Work out the finished part from the listing and answer in its coordinate system (mm). A direction names the side the tool comes from. Give positions to 0.01 mm unless a question says otherwise; leave off trailing zeros. Loops run counter-clockwise (first coordinate to the right, second up) from the corner with the lowest first, then second, coordinate; pieces in that order, holes last. Notation, with made-up numbers: M 51.25,13 L 65.25,13 A13 cw 65.25,36 Z; hole C 82.25,-33 d2. An arc over 180 degrees is marked long. Answer in a Markdown table with one row per item. Add a question column.
from build123d import *

# Parameters (mm, degrees)
SKETCH1_W                  = 40
SKETCH1_H                  = 25
BOSS_EXTRUDE1_DEPTH        = 2
SKETCH2_W                  = 5
SKETCH2_H                  = 20
BOSS_EXTRUDE2_DEPTH        = 10
SKETCH4_W                  = 19.965035534
SKETCH4_H                  = 6
BOSS_EXTRUDE3_DEPTH        = 5
SKETCH5_R                  = 1
CUT_EXTRUDE2_DEPTH         = 5
SKETCH6_W                  = 4
SKETCH6_H                  = 5
BOSS_EXTRUDE4_DEPTH        = 10
SKETCH8_W                  = 5
SKETCH8_H                  = 4
BOSS_EXTRUDE5_DEPTH        = 10
SKETCH9_W                  = 4
SKETCH9_H                  = 5
BOSS_EXTRUDE6_DEPTH        = 45
SKETCH12_W                 = 18
SKETCH12_H                 = 4
BOSS_EXTRUDE8_DEPTH        = 4
SKETCH13_W                 = 5
SKETCH13_H                 = 4
BOSS_EXTRUDE9_DEPTH        = 26
SKETCH14_W                 = 18
SKETCH14_H                 = 4
BOSS_EXTRUDE10_DEPTH       = 6
SKETCH16_W                 = 5.988277512
SKETCH16_H                 = 18
BOSS_EXTRUDE11_DEPTH       = 5
SKETCH15_R                 = 1
CUT_EXTRUDE3_DEPTH         = 6
SKETCH17_R                 = 3
CUT_EXTRUDE5_DEPTH         = 6
SKETCH24_W                 = 8
SKETCH24_H                 = 18.5
BOSS_EXTRUDE18_DEPTH       = 4
BOSS_EXTRUDE20_START       = -1
SKETCH20_R                 = 5
SKETCH20_R_2               = 3
BOSS_EXTRUDE20_DEPTH       = 1
BOSS_EXTRUDE21_OUTLINE_R   = 2.998308623
BOSS_EXTRUDE21_OUTLINE_R_2 = 1.5
BOSS_EXTRUDE21_DEPTH       = 1
SKETCH27_R                 = 5
SKETCH27_R_2               = 2.75
BOSS_EXTRUDE22_DEPTH       = 2
SKETCH28_R                 = 2.75
CUT_EXTRUDE10_DEPTH        = 10
SKETCH29_R                 = 5
BOSS_EXTRUDE23_DEPTH       = 5


# Read off the part's stored shape, not the designer's step: Boss-Extrude21
with BuildPart() as part:
    # Sketch1 → Boss-Extrude1 (new body)
    with BuildSketch(Plane(origin=(0, 0, 0), x_dir=(1, 0, 0), z_dir=(0, 1, 0))):
        Rectangle(SKETCH1_W, SKETCH1_H)
    extrude(amount=BOSS_EXTRUDE1_DEPTH)

    # Sketch2 → Boss-Extrude2 (add)
    with BuildSketch(Plane(origin=(0, 2, 0), x_dir=(1, 0, 0), z_dir=(0, 1, 0))):
        with Locations((4.5, 0)):
            Rectangle(SKETCH2_W, SKETCH2_H)
    extrude(amount=BOSS_EXTRUDE2_DEPTH)

    # Sketch4 → Boss-Extrude3 (add)
    with BuildSketch(Plane(origin=(7, 0, 0), x_dir=(0, 0, -1), z_dir=(1, 0, 0))):
        with Locations((-0.017482233, 9)):
            Rectangle(SKETCH4_W, SKETCH4_H)
    extrude(amount=-BOSS_EXTRUDE3_DEPTH)

    # Sketch5 → Cut-Extrude2 (cut)
    with BuildSketch(Plane(origin=(7, 0, 0), x_dir=(0, 0, -1), z_dir=(1, 0, 0))):
        with Locations((5, 7.5)):
            Circle(SKETCH5_R)
        with Locations((-5, 7.5)):
            Circle(SKETCH5_R)
    extrude(amount=-CUT_EXTRUDE2_DEPTH, mode=Mode.SUBTRACT)

    # Sketch6 → Boss-Extrude4 (add)
    with BuildSketch(Plane(origin=(0, 2, 0), x_dir=(1, 0, 0), z_dir=(0, 1, 0))):
        with Locations((-11.527661753, -6.5)):
            Rectangle(SKETCH6_W, SKETCH6_H)
        with Locations((-11.527661753, 6.5)):
            Rectangle(SKETCH6_W, SKETCH6_H)
    extrude(amount=BOSS_EXTRUDE4_DEPTH)

    # Sketch8 → Boss-Extrude5 (add)
    with BuildSketch(Plane.ZY.offset(13.527661753)):
        with Locations((-6.5, 10)):
            Rectangle(SKETCH8_W, SKETCH8_H)
    boss_extrude5 = extrude(amount=BOSS_EXTRUDE5_DEPTH)

    # Mirror1: Boss-Extrude5 across plane
    add(boss_extrude5.mirror(Plane(origin=(0, 0, 0), x_dir=(1, 0, 0), z_dir=(0, 0, -1))))

    # Sketch9 → Boss-Extrude6 (add)
    with BuildSketch(Plane(origin=(0, 12, 0), x_dir=(1, 0, 0), z_dir=(0, 1, 0))):
        with Locations((-21.527661753, 6.5)):
            Rectangle(SKETCH9_W, SKETCH9_H)
    boss_extrude6 = extrude(amount=BOSS_EXTRUDE6_DEPTH)

    # Mirror2: Boss-Extrude5 across plane
    add(boss_extrude5.mirror(Plane(origin=(0, 0, 0), x_dir=(1, 0, 0), z_dir=(0, 0, -1))))

    # Mirror3: Boss-Extrude6 across plane
    add(boss_extrude6.mirror(Plane(origin=(0, 0, 0), x_dir=(1, 0, 0), z_dir=(0, 0, -1))))

    # Sketch12 → Boss-Extrude8 (add)
    with BuildSketch(Plane.ZY.offset(23.527661753)):
        with Locations((0, 55)):
            Rectangle(SKETCH12_W, SKETCH12_H)
        with Locations((0, 10)):
            Rectangle(SKETCH12_W, SKETCH12_H)
        with Locations((0, 32.5)):
            Rectangle(SKETCH12_W, SKETCH12_H)
    extrude(amount=-BOSS_EXTRUDE8_DEPTH)

    # Sketch13 → Boss-Extrude9 (add)
    with BuildSketch(Plane(origin=(-19.527661753, 0, 0), x_dir=(0, 0, -1), z_dir=(1, 0, 0))):
        with Locations((-6.5, 55)):
            Rectangle(SKETCH13_W, SKETCH13_H)
        with Locations((6.5, 55)):
            Rectangle(SKETCH13_W, SKETCH13_H)
    extrude(amount=BOSS_EXTRUDE9_DEPTH)

    # Sketch14 → Boss-Extrude10 (add)
    with BuildSketch(Plane(origin=(6.472338247, 0, 0), x_dir=(0, 0, -1), z_dir=(1, 0, 0))):
        with Locations((0, 55)):
            Rectangle(SKETCH14_W, SKETCH14_H)
    extrude(amount=-BOSS_EXTRUDE10_DEPTH)

    # Sketch16 → Boss-Extrude11 (add)
    with BuildSketch(Plane(origin=(0, 57, 0), x_dir=(1, 0, 0), z_dir=(0, 1, 0))):
        with Locations((3.478199491, 0)):
            Rectangle(SKETCH16_W, SKETCH16_H)
    extrude(amount=BOSS_EXTRUDE11_DEPTH)

    # Sketch15 → Cut-Extrude3 (cut)
    with BuildSketch(Plane(origin=(6.472338247, 0, 0), x_dir=(0, 0, -1), z_dir=(1, 0, 0))):
        with Locations((-5, 57.5)):
            Circle(SKETCH15_R)
        with Locations((5, 57.5)):
            Circle(SKETCH15_R)
    extrude(amount=-CUT_EXTRUDE3_DEPTH, mode=Mode.SUBTRACT)

    # Sketch17 → Cut-Extrude5 (cut)
    with BuildSketch(Plane.XZ):
        with Locations(Location((0, 0, 0), (0, 0, 270))):
            Circle(SKETCH17_R)
    extrude(amount=-CUT_EXTRUDE5_DEPTH, mode=Mode.SUBTRACT)

    # Sketch24 → Boss-Extrude18 (add)
    with BuildSketch(Plane.ZY.offset(23.527661753)):
        with Locations((0, 43.75)):
            Rectangle(SKETCH24_W, SKETCH24_H)
    extrude(amount=-BOSS_EXTRUDE18_DEPTH)

    # Sketch20 → Boss-Extrude20 (add)
    with BuildSketch(Plane(origin=(0, 3, 0), x_dir=(1, 0, 0), z_dir=(0, 1, 0)).offset(BOSS_EXTRUDE20_START)):
        Circle(SKETCH20_R)
        with Locations(Location((0, 0, 0), (0, 0, 90))):
            Circle(SKETCH20_R_2, mode=Mode.SUBTRACT)
    extrude(amount=BOSS_EXTRUDE20_DEPTH)

    # Boss-Extrude21 outline → Boss-Extrude21 (add)
    # profile 1 of 2: a face of its own
    with BuildSketch(Plane(origin=(0, 3, 0), x_dir=(1, 0, 0), z_dir=(0, 1, 0))):
        with BuildLine():
            ThreePointArc((2, -2.236067977), (-3, 0), (2, 2.236067977))
            Line((2, 2.236067977), (2, 4.582575695))
            ThreePointArc((2, 4.582575695), (-5, 0), (2, -4.582575695))
            Line((2, -4.582575695), (2, -2.236067977))
        make_face()
    # profile 2 of 2: a face of its own
    with BuildSketch(Plane(origin=(0, 3, 0), x_dir=(1, 0, 0), z_dir=(0, 1, 0))):
        Circle(BOSS_EXTRUDE21_OUTLINE_R)
        Circle(BOSS_EXTRUDE21_OUTLINE_R_2, mode=Mode.SUBTRACT)
    extrude(amount=BOSS_EXTRUDE21_DEPTH)

    # Sketch27 → Boss-Extrude22 (add)
    with BuildSketch(Plane(origin=(0, 4, 0), x_dir=(1, 0, 0), z_dir=(0, 1, 0))):
        Circle(SKETCH27_R)
        with Locations(Location((0, 0, 0), (0, 0, 43.341758227))):
            Circle(SKETCH27_R_2, mode=Mode.SUBTRACT)
    extrude(amount=BOSS_EXTRUDE22_DEPTH)

    # Sketch28 → Cut-Extrude10 (cut)
    with BuildSketch(Plane(origin=(0, 6, 0), x_dir=(1, 0, 0), z_dir=(0, 1, 0))):
        with Locations(Location((0, 0, 0), (0, 0, 43.341758227))):
            Circle(SKETCH28_R)
    extrude(amount=CUT_EXTRUDE10_DEPTH, mode=Mode.SUBTRACT)

    # Sketch29 → Boss-Extrude23 (add)
    with BuildSketch(Plane.ZY.offset(23.527661753)):
        with Locations((-0.05, 43.4)):
            Circle(SKETCH29_R)
    extrude(amount=BOSS_EXTRUDE23_DEPTH)


solid = part.part
(1) Each of these flat-tipped pins is pushed along its axis until it touches: P1, Ø2.5, axis at y = 4, z = 6.5, coming from the -X side; P2, Ø1, axis at y = 36.5, z = 2.5, coming from the +X side; P3, Ø1.6, axis at y = 57.5, z = -5, coming from the +X side. Where does it stop, or does it pass through?
(2) Section B-B, the plane z = 7 is taken. Determine the outline of the cut face in (x, y).
(3) The mould has two halves that part along Y. Classify faces 1 (the face through (1.3, 3, 1.3)), 2 (the face through (-13, 8, 4)), 3 (the face through (-25.99, 38.52, -1.13)), 4 (the face through (4.54, 8.49, -4.87)): pulls with the +Y half, pulls with the -Y half, needs draft (parallel to the pull), parting line crosses it, or undercut.
(4) Section D-D, the plane y = 37.5 is taken. Determine the outline of the cut face in (x, z), and give its area (3 significant figures).
(5) Section A-A, the plane y = 10.5 is taken. Determine the outline of the cut face in (x, z).
(6) Section C-C, the plane x = -24.5 is taken. Determine the outline of the cut face in (y, z).
(7) Which of the six approach directions +Z, -Z, +X, -X, +Y, -Y give full straight-line access (tool end or side, diameter ignored) to faces 5 (the face through (-22, 30.5, 0)), 6 (the face through (-9.528, 7, 7)), 7 (the face through (-20, 8, 0)), 8 (the face through (3.51, 58.34, -5.54))?
(8) Consider line 1 along Y through (x, z) = (5.85, 5); line 2 along Z through (x, y) = (5, 57.5); line 3 along X through (y, z) = (9, -2). Determine where each line is inside the solid, lowest interval first. Write a range as from..to.
Numbers:
| question | item | result |
|---|---|---|
| 1 | P1 | stops at x = -13.53 |
| 1 | P2 | stops at x = -19.53 |
| 1 | P3 | stops at x = 0.47 |
| 2 | outline | M -23.53,8 L -13.53,8 L -13.53,2 L -20,2 L -20,0 L 20,0 L 20,2 L 7,2 L 7,12 L 2,12 L 2,2 L -9.53,2 L -9.53,12 L -19.53,12 L -19.53,53 L 6.47,53 L 6.47,62 L 0.48,62 L 0.48,57 L -23.53,57 Z |
| 3 | face 1 | pulls with the -Y half |
| 3 | face 2 | needs draft |
| 3 | face 3 | parting line crosses it |
| 3 | face 4 | undercut |
| 4 | outline | M -23.53,-9 L -19.53,-9 L -19.53,9 L -23.53,9 Z |
| 4 | area | 72.0 mm² |
| 5 | outline | M -23.53,-9 L -9.53,-9 L -9.53,-4 L -19.53,-4 L -19.53,4 L -9.53,4 L -9.53,9 L -23.53,9 Z; M 2,-10 L 7,-10 L 7,10 L 2,10 L 2,1.89 A2.75 cw 2,-1.89 Z |
| 6 | outline | C 43.4,-0.05 d10 |
| 7 | face 5 | +X, -X |
| 7 | face 6 | +Z, -Z |
| 7 | face 7 | +Z, -Z, -X |
| 7 | face 8 | +X |
| 8 | line 1 | y = 0..6.5, 8.5..12, 53..56.5, 58.5..62 |
| 8 | line 2 | z = -9..-6, -4..4, 6..9 |
| 8 | line 3 | x = -23.53..-19.53, 2..7 |
